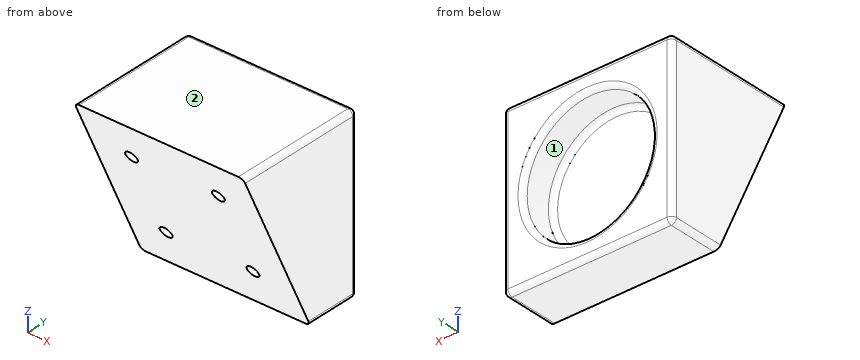
Autodesk Inventor part; units mm, degrees
ref_plane "YZ Plane" through (0, 0, 0) normal (1, 0, 0) x (0, 1, 0)
ref_plane "XZ Plane" through (0, 0, 0) normal (0, 1, 0) x (-1, 0, 0)
ref_plane "XY Plane" through (0, 0, 0) normal (0, 0, 1) x (1, 0, 0)
sketch "Sketch1" plane through (0, 0, 0) normal (1, 0, 0) x (0, 1, 0)
  line L0 (0, 0) -> (-50.3379, 107.95)
  line L1 (-50.3379, 107.95) -> (34.925, 107.95)
  line L2 (34.925, 107.95) -> (34.925, 0)
  line L3 (34.925, 0) -> (0, 0)
  line L4 (0, 0) -> (0, 107.95) construction
  dimension "tilt" = 25
  dimension "baseDepth" = 107.95
  dimension "holderHeight" = 34.925
extrude "Extrusion1" add sketch "Sketch1" along normal mid plane 107.95
sketch "Sketch2" plane through (-53.975, 34.925, 107.95) normal (0, 1, 0) x (1, 0, 0)
  line L0 (107.95, 0) -> (0, 0) construction
  line L1 (107.95, 0) -> (107.95, 107.95) construction
  line L2 (0, 0) -> (107.95, 107.95) construction
  line L3 (0, 107.95) -> (107.95, 107.95) construction
  line L4 (0, 107.95) -> (107.95, 0) construction
  circle A0 centre (53.975, 53.975) radius 41.275
  point P0 (53.975, 107.95)
  dimension "d5" = 82.55
extrude "Extrusion2" cut sketch "Sketch2" against normal blind 22.225
sketch "Sketch4" plane through (-53.975, 0, 0) normal (0, -0.9063078, -0.4226183) x (1, 0, 0)
  line L0 (107.95, 119.1096) -> (107.95, 0) construction
  line L1 (107.95, 119.1096) -> (0, 119.1096) construction
  line L2 (107.95, 0) -> (0, 119.1096) construction
  line L3 (0, 0) -> (107.95, 0) construction
  line L4 (0, 0) -> (107.95, 119.1096) construction
  circle A0 centre (53.975, 59.5548) radius 41.275 construction
  ellipse E0 centre (53.975, 43.5507) end of major axis (12.7, 43.5507) minor radius 37.4079
  point P0 (53.975, 0)
  point P1 (81.6929, 90.1382)
  point P2 (81.6929, 28.9715)
  point P3 (26.2571, 28.9715)
  point P4 (26.2571, 90.1382)
  dimension "d14" = 82.55
hole "Hole2" at (27.7179, -38.094, 81.6929) at (27.7179, -12.2439, 26.2571) at (-27.7179, -12.2439, 26.2571) at (-27.7179, -38.094, 81.6929) direction (0, 0.9063078, 0.4226183) diameter 7.7978 depth 22.225 tip angle 118
fillet "Fillet1" radius 3.175 2 edges at (-41.275, 34.925, 53.975) (-41.275, 12.7, 53.975)
fillet "Fillet2" radius 3.175 4 edges at (0, 34.925, 107.95) (-53.975, 34.925, 53.975) (0, 34.925, 0) (53.975, 34.925, 53.975)
fillet "Fillet3" radius 3.175 8 edges at (-53.0451, 33.9951, 107.0201) (-53.975, -9.294, 107.95) (53.0451, 33.9951, 107.0201) (53.975, -9.294, 107.95) (53.0451, 33.9951, 0.9299) (53.975, 15.875, 0) (-53.0451, 33.9951, 0.9299) (-53.975, 15.875, 0)
equation "\"d5\" = cupDiam"
equation "\"d6\" = cupDepth"
equation "\"d14\" = cupDiam"
equation "\"d27\" = threadHoleDepth"
equation "\"d29\" = filet"
equation "\"d30\" = filet"
equation "\"d31\" = filet"
equation "\"cupDiam\" = 82.55"
equation "\"cupDepth\" = 22.225"
equation "\"threadHoleDepth\" = 22.225"
equation "\"filet\" = 3.175"
properties part number "ChickenCupHolder"
The model under review builds one solid part; all positions refer to its coordinate system, in mm. Face numbers are marked on the shaded views. A direction names the side the tool comes from. Give positions to 0.01 mm unless a question says otherwise; leave off trailing zeros. Write each loop counter-clockwise with the first axis right and the second up, starting at its lowest first coordinate (ties: lowest second). Pieces come first, ordered by that corner, then holes. Notation, with made-up numbers: (75.25, 33) - (81.25, 33) arc R18 cw to (81.25, 50) - close; hole circle Ø10 at (-33.5, 17.25). An arc over 180 degrees is marked (long way). Answer in a Markdown table with one row per item. Add a question column.
1. Wall thickness on line 1 along Z through (x, y) = (0, 20); line 2 along X through (y, z) = (24.5, 61) (3 decimals); line 3 along X through (y, z) = (25, 32) (3 decimals): over which ranges is each line inside the solid? List them lowest first. Write a range as [from, to].
2. We need section B-B on x = 0. Write out the cut boundary in (y, z) (3 decimals).
3. We need section D-D on y = -44. Write out the cut boundary in (x, z) (3 decimals), then the cut area to 3 significant figures.
4. We need section A-A on y = 18. Write out the cut boundary in (x, z) (3 decimals), then the cut area to 3 significant figures.
5. We need section C-C on z = 7. Write out the cut boundary in (x, y) (3 decimals).
6. Insertion check: P1, Ø12, axis at x = -17.5, z = 54, coming from the +Y side; P2, Ø2, axis at x = 25, z = 71.5, coming from the -Y side; P3, Ø10, axis at x = -32.5, y = -22, coming from the -Z side. Each pin has a flat end and moves straight along its axis. Give the tip position at first contact, or say it passes through.
7. Tool access review of the marked faces 1 and 2: name each direction out of +Z, -Z, +X, -X, +Y, -Y from which nothing blocks a thin tool from reaching the whole face with its end or side.
Ans:
| question | item | result |
|---|---|---|
| 1 | line 1 | z = [0, 12.7], [95.25, 107.95] |
| 1 | line 2 | x = [-53.975, -40.673], [40.673, 53.975] |
| 1 | line 3 | x = [-53.975, -34.939], [34.939, 53.975] |
| 2 | outline | (-50.338, 107.95) - (0, 0) - (31.75, 0) arc R3.175 ccw to (34.925, 3.175) - (34.925, 9.525) arc R3.175 ccw to (31.75, 12.7) - (15.875, 12.7) arc R3.175 cw to (12.7, 15.875) - (12.7, 92.075) arc R3.175 cw to (15.875, 95.25) - (31.75, 95.25) arc R3.175 ccw to (34.925, 98.425) - (34.925, 104.775) arc R3.175 ccw to (31.75, 107.95) - close |
| 3 | outline | (-53.975, 94.358) - (53.975, 94.358) - (53.975, 104.775) arc R3.175 ccw to (50.8, 107.95) - (-50.8, 107.95) arc R3.175 ccw to (-53.975, 104.775) - close |
| 3 | area | 1,460 mm^2 |
| 4 | outline | (-53.975, 3.175) arc R3.175 ccw to (-50.8, 0) - (50.8, 0) arc R3.175 ccw to (53.975, 3.175) - (53.975, 104.775) arc R3.175 ccw to (50.8, 107.95) - (-50.8, 107.95) arc R3.175 ccw to (-53.975, 104.775) - close; hole circle Ø82.55 at (0, 53.975) |
| 4 | area | 6,290 mm^2 |
| 5 | outline | (-53.975, -3.264) - (53.975, -3.264) - (53.975, 31.75) arc R3.175 ccw to (50.8, 34.925) - (-50.8, 34.925) arc R3.175 ccw to (-53.975, 31.75) - close |
| 6 | P1 | stops at y = 12.7 |
| 6 | P2 | stops at y = -33.81 |
| 6 | P3 | stops at z = 36.46 |
| 7 | face 1 | +Y |
| 7 | face 2 | +Z, +X, -X, +Y, -Y |
